The listing builds one solid part. Answer for the finished solid, in the listing's coordinates (mm). Face numbers are marked on the shaded views. A direction names the side the tool comes from. Give positions to 0.01 mm unless a question says otherwise; leave off trailing zeros. Write each loop counter-clockwise with the first axis right and the second up, starting at its lowest first coordinate (ties: lowest second). Pieces come first, ordered by that corner, then holes. Notation, with made-up numbers: (28.5, 64.25) -> (63.5, 64.25) arc R32 cw to (63.5, 96.25) -> close; hole circle Ø11 at (-29, -14.5). An arc over 180 degrees is marked (long way). One line per question, with ' | ' between items.
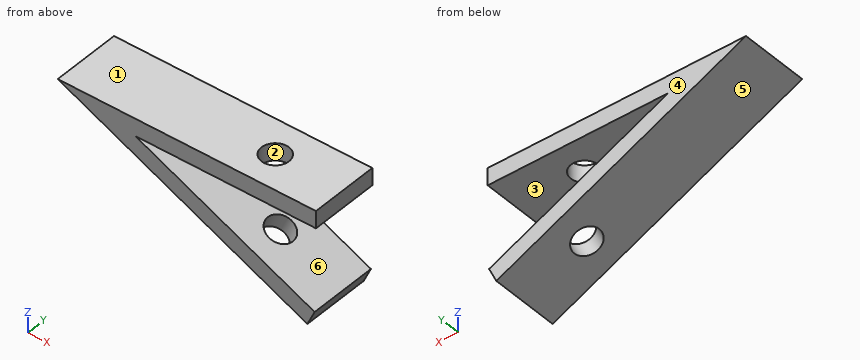
from build123d import *

# Parameters (mm, degrees)
BOSS_EXTRUDE1_DEPTH = 20
SKETCH2_R           = 4
CUT_EXTRUDE2_DEPTH  = 5
SKETCH3_R           = 4
CUT_EXTRUDE3_DEPTH  = 5


with BuildPart() as part:
    # Sketch1 → Boss-Extrude1 (new body)
    with BuildSketch(Plane(origin=(0, 0, 0), x_dir=(1, 0, 0), z_dir=(0, 1, 0))):
        Polygon((0, 0), (37.679677005, 0), (37.679677005, 5), (-14.766780477, 5), (37.297391276, 29.277922004), (35.184299968, 33.809460939), (-37.320322995, 0), align=None)
    extrude(amount=BOSS_EXTRUDE1_DEPTH)

    # Sketch2 → Cut-Extrude2 (cut)
    with BuildSketch(Plane(origin=(-6.665640892, 0, -14.294513023), x_dir=(-0.9063077870366526, 0, 0.42261826174069417), z_dir=(-0.42261826174069417, 0, -0.9063077870366526))):
        with Locations((-26.176300655, 10)):
            Circle(SKETCH2_R)
    extrude(amount=-CUT_EXTRUDE2_DEPTH, mode=Mode.SUBTRACT)

    # Sketch3 → Cut-Extrude3 (cut)
    with BuildSketch(Plane.XY):
        with Locations((17.679677005, 10)):
            Circle(SKETCH3_R)
    extrude(amount=-CUT_EXTRUDE3_DEPTH, mode=Mode.SUBTRACT)


solid = part.part
Item 1: Find section D-D (z = -8). Write down the section's boundary in (x, y), then the cut area to 3 significant figures.
Answers below:
outline: (-20.16, 0) -> (-8.33, 0) -> (-8.33, 20) -> (-20.16, 20) -> close | area: 237 mm²
Item 2: Flat-ended cylindrical pins translate along their axes: pin 1 (10 mm diameter, centred on x = 6, y = 4.5, fed in from +Z); pin 2 (6 mm diameter, centred on y = 14, z = -5, fed in from -X); pin 3 (3 mm diameter, centred on y = 6, z = -8.5, fed in from +X); pin 4 (12 mm diameter, centred on y = 16.5, z = -24.5, fed in from -X). Find the tip coordinate at first contact, or state that the pin passes through.
Answers below:
pin 1: z = 0 | pin 2: x = -33.03 | pin 3: x = -4.04 | pin 4: x = 2.35
Item 3: Consider line 1 (Z direction, x = 28, y = 8); line 2 (Z direction, x = -4.5, y = 5); line 3 (X direction, y = 9.75, z = -1.5). Determine where each line is inside the solid, lowest interval first. Write a range as [from, to].
Answers below:
line 1: [-30.46, -24.94], [-5, 0] | line 2: [-15.3, -9.79], [-5, 0] | line 3: [-34.1, 13.69], [21.67, 37.68]
Item 4: A tool of negligible diameter and unlimited length cuts with its end or side. For the marked faces 1, 2 and 3, from which of +Z, -Z, +X, -X, +Y, -Y can it reach the whole face along a straight path? Write none if from no direction.
Answers below:
face 1: +Z, +X, -X, +Y, -Y | face 2: +Z | face 3: +X, +Y, -Y
Item 5: Determine the mould class of the marked faces 4, 5 and 6 for opening direction Z: pulls with the +Z half, pulls with the -Z half, needs draft (parallel to the pull), parting line crosses it, or undercut.
Answers below:
face 4: needs draft | face 5: pulls with the -Z half | face 6: undercut
Item 6: Find section B-B (x = 25.5). Write down the section's boundary in (y, z).
Answers below:
outline: (0, -29.29) -> (20, -29.29) -> (20, -23.78) -> (0, -23.78) -> close; (0, -5) -> (20, -5) -> (20, 0) -> (0, 0) -> close
Item 7: Find section A-A (y = 10). Write down the section's boundary in (x, z).
Answers below:
outline: (-37.32, 0) -> (13.43, -23.67) -> (15.55, -19.14) -> (-14.77, -5) -> (13.68, -5) -> (13.68, 0) -> close; (20.68, -27.05) -> (35.18, -33.81) -> (37.3, -29.28) -> (22.8, -22.52) -> close; (21.68, -5) -> (37.68, -5) -> (37.68, 0) -> (21.68, 0) -> close
Item 8: Find section C-C (y = 17). Write down the section's boundary in (x, z).
Answers below:
outline: (-37.32, 0) -> (35.18, -33.81) -> (37.3, -29.28) -> (-14.77, -5) -> (37.68, -5) -> (37.68, 0) -> close
